Geometry: final body of the model. Coordinates: model frame, mm. Face numbers are marked on the shaded views. A direction names the side the tool comes from. Give positions to 0.01 mm unless a question says otherwise; leave off trailing zeros. Write each loop counter-clockwise with the first axis right and the second up, starting at its lowest first coordinate (ties: lowest second). Pieces come first, ordered by that corner, then holes.
Q1. Pin query (flat end, axial travel): pin 1 (5 mm diameter, centred on x = 1.27, y = 0, fed in from +Z); pin 2 (3 mm diameter, centred on x = 4.5, z = 6, fed in from +Y). Return the tip coordinate at first contact, or that it passes through.
Q2. Cut plane A-A on y = 0. Return the cut outline in (x, z) (1 decimal), plus the area to 3 significant figures.
Q3. Cut plane D-D on x = 8.5. Return the cut outline in (y, z) (3 decimals), plus the area to 3 significant figures.
Q4. Draft query along Y for the marked faces 3, 4 and 5. Return one class per face: pulls with the +Y half, pulls with the -Y half, needs draft (parallel to the pull), parting line crosses it, or undercut.
Q5. Reachability of the marked faces 1 and 2 from +Z, -Z, +X, -X, +Y, -Y: full face, straight path, thin tool, end or side. Return the list, or none.
Q6. Cut plane C-C on z = 2.75. Return the cut outline in (x, y), plus the area to 3 significant figures.
Q7. Line query: L1, parallel to X at y = 0, z = 1.5; L2, parallel to Y at x = 1.25, z = 1.5; L3, parallel to X at y = -1.25, z = 0.5. Output: solid intervals per line, ascending.
Q8. Cut plane B-B on x = -3.25. Return the cut outline in (y, z) (3 decimals).
```python
from build123d import *

# Parameters (mm, degrees)
BOSS_EXTRUDE1_DEPTH     = 3.175
SKETCH4_R               = 6.31825
BOSS_EXTRUDE2_DEPTH     = 3.96875
CUT_EXTRUDE1_DEPTH      = 16.014259108
CUT_EXTRUDE1_DEPTH_BACK = 16.014259108
SKETCH2_R               = 0.9
CUT_EXTRUDE2_DEPTH      = 16.014259108
CUT_EXTRUDE2_DEPTH_BACK = 3.81
SKETCH3_R               = 1.7145


with BuildPart() as part:
    # Sketch1 → Boss-Extrude1 (new body)
    with BuildSketch(Plane.XY):
        with BuildLine():
            Line((0, 8.89), (2.54, 8.89))
            ThreePointArc((2.54, 8.89), (11.43, 0), (2.54, -8.89))
            Line((2.54, -8.89), (0, -8.89))
            ThreePointArc((0, -8.89), (-8.89, 0), (0, 8.89))
        make_face()
    extrude(amount=BOSS_EXTRUDE1_DEPTH)

    # Sketch4 → Boss-Extrude2 (add)
    with BuildSketch(Plane.XY.offset(3.175)):
        with Locations((2.54, 0)):
            Circle(SKETCH4_R)
    extrude(amount=BOSS_EXTRUDE2_DEPTH)

    # Sketch2 → Cut-Extrude1 (cut, two sides: drawn at the far end of the back side and taken through both)
    with BuildSketch(Plane.XY.offset(3.175).offset(-CUT_EXTRUDE1_DEPTH_BACK)):
        with Locations((-3.81, 0)):
            Circle(SKETCH2_R)
        with BuildLine():
            Line((2.835761157, 2.159), (-0.295761157, 2.159))
            ThreePointArc((-0.295761157, 2.159), (1.27, -2.667), (2.835761157, 2.159))
        make_face()
    extrude(amount=CUT_EXTRUDE1_DEPTH + CUT_EXTRUDE1_DEPTH_BACK, mode=Mode.SUBTRACT)

    # Sketch3 → Cut-Extrude2 (cut, two sides: drawn at the far end of the back side and taken through both)
    with BuildSketch(Plane.XY.offset(3.175).offset(-CUT_EXTRUDE2_DEPTH_BACK)):
        with Locations(Location((-3.81, 0, 0), (0, 0, 278.828200895))):
            Circle(SKETCH3_R)
    extrude(amount=CUT_EXTRUDE2_DEPTH + CUT_EXTRUDE2_DEPTH_BACK, mode=Mode.SUBTRACT)


solid = part.part
```
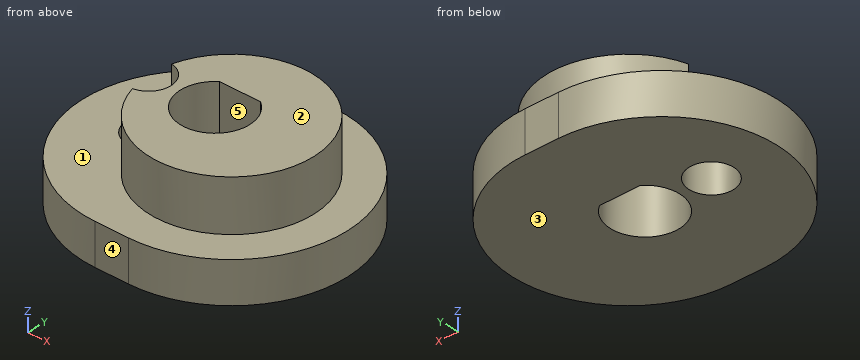
Data:
1. pin 1: stops at z = 7.14
1. pin 2: stops at y = 6.3
2. outline: (-8.9, 0) - (-5.5, 0) - (-5.5, 3.2) - (-8.9, 3.2) - close; (-2.1, 0) - (-1.4, 0) - (-1.4, 7.1) - (-2.1, 7.1) - close; (3.9, 0) - (11.4, 0) - (11.4, 3.2) - (8.9, 3.2) - (8.9, 7.1) - (3.9, 7.1) - close
2. area: 59.0 mm2
3. outline: (-6.596, 0) - (6.596, 0) - (6.596, 3.175) - (2.097, 3.175) - (2.097, 7.144) - (-2.097, 7.144) - (-2.097, 3.175) - (-6.596, 3.175) - close
3. area: 58.5 mm2
4. face 3: needs draft
4. face 4: pulls with the -Y half
4. face 5: undercut
5. face 1: +Z
5. face 2: +Z, +X, -X, +Y, -Y
6. outline: (0, -8.89) - (2.54, -8.89) arc R8.89 ccw to (2.54, 8.89) - (0, 8.89) arc R8.89 ccw to start; hole circle Ø3.43 at (-3.81, 0); hole (-0.3, 2.16) arc R2.67 ccw (long way) to (2.84, 2.16) - close
6. area: 263 mm2
7. L1: x = -8.89 to -5.52, -2.1 to -1.4, 3.94 to 11.43
7. L2: y = -8.89 to -2.67, 2.16 to 8.89
7. L3: x = -8.8 to -4.98, -2.64 to -1.09, 3.63 to 11.34
8. outline: (-8.275, 0) - (-1.62, 0) - (-1.62, 7.144) - (-2.529, 7.144) - (-2.529, 3.175) - (-8.275, 3.175) - close; (1.62, 0) - (8.275, 0) - (8.275, 3.175) - (2.529, 3.175) - (2.529, 7.144) - (1.62, 7.144) - close
